CAD build for the part. Positions are in the model's coordinates, mm. Give positions to 0.01 mm unless a question says otherwise; leave off trailing zeros. Loops run counter-clockwise (first coordinate to the right, second up) from the corner with the lowest first, then second, coordinate; pieces in that order, holes last.
Item 1: Probe probe 1 along Y at (x, z) = (-1, 200); probe 2 along X at (y, z) = (-3.5, 490.5); probe 3 along X at (y, z) = (23, 372). List the from-to ranges inside material, lowest first.
Item 2: Saw through at A-A on y = -4. Give the cut face in (x, z).
Item 3: Drop flat-ended pins along their axis: P1, Ø3, axis at x = 8, z = 513, coming from the +Y side; P2, Ø8, axis at x = 0, z = 31.75, coming from the -Y side; P3, Ø4.5, axis at x = 0, z = 539.75, coming from the -Y side. Give the stop position or say it passes through.
from build123d import *

# Parameters (mm, degrees)
EXTRUDE_THIN1_DEPTH               = 571.5
F_10_CLEARANCE_HOLE1_D            = 5.1054
F_3_16_0_195_DIAMETER_HOLE1_D     = 4.953
F_3_16_0_195_DIAMETER_HOLE1_DEPTH = 1.5875


with BuildPart() as part:
    # Sketch1 → Extrude-Thin1 (new body)
    with BuildSketch(Plane.XY):
        with BuildLine():
            Line((-12.7, 19.05), (-12.7, -19.05))
            ThreePointArc((-12.7, -19.05), (-10.840128061, -23.540128061), (-6.35, -25.4))
            Line((-6.35, -25.4), (6.35, -25.4))
            ThreePointArc((6.35, -25.4), (10.840128061, -23.540128061), (12.7, -19.05))
            Line((12.7, -19.05), (12.7, 19.05))
            ThreePointArc((12.7, 19.05), (10.840128061, 23.540128061), (6.35, 25.4))
            Line((6.35, 25.4), (-6.35, 25.4))
            ThreePointArc((-6.35, 25.4), (-10.840128061, 23.540128061), (-12.7, 19.05))
        make_face()
        with BuildLine():
            Line((-11.1125, 19.05), (-11.1125, -19.05))
            ThreePointArc((-11.1125, -19.05), (-9.717596045, -22.417596045), (-6.35, -23.8125))
            Line((-6.35, -23.8125), (6.35, -23.8125))
            ThreePointArc((6.35, -23.8125), (9.717596045, -22.417596045), (11.1125, -19.05))
            Line((11.1125, -19.05), (11.1125, 19.05))
            ThreePointArc((11.1125, 19.05), (9.717596045, 22.417596045), (6.35, 23.8125))
            Line((6.35, 23.8125), (-6.35, 23.8125))
            ThreePointArc((-6.35, 23.8125), (-9.717596045, 22.417596045), (-11.1125, 19.05))
        make_face(mode=Mode.SUBTRACT)
    extrude(amount=EXTRUDE_THIN1_DEPTH)

    # #10 Clearance Hole1 (through all)
    with Locations(Plane(origin=(0, 25.4, 565.15), x_dir=(0, 0, 1), z_dir=(0, 1, 0))):
        with Locations((0, 0), (-558.8, 0), (-533.4, 0), (-508, 0), (-25.4, 0), (-50.8, 0)):
            Hole(F_10_CLEARANCE_HOLE1_D / 2)

    # 3/16 (0.195) Diameter Hole1
    with Locations(Plane(origin=(0, 25.4, 0), x_dir=(1, 0, 0), z_dir=(0, 1, 0))):
        with Locations((-3.175, -82.55), (3.175, -107.95), (-3.175, -133.35), (3.175, -158.75), (-3.175, -184.15), (3.175, -209.55), (-3.175, -234.95), (3.175, -260.35), (-3.175, -285.75), (3.175, -311.15), (-3.175, -336.55), (3.175, -361.95), (-3.175, -387.35), (3.175, -412.75), (-3.175, -438.15), (3.175, -463.55), (-3.175, -488.95)):
            Hole(F_3_16_0_195_DIAMETER_HOLE1_D / 2, depth=F_3_16_0_195_DIAMETER_HOLE1_DEPTH)


solid = part.part
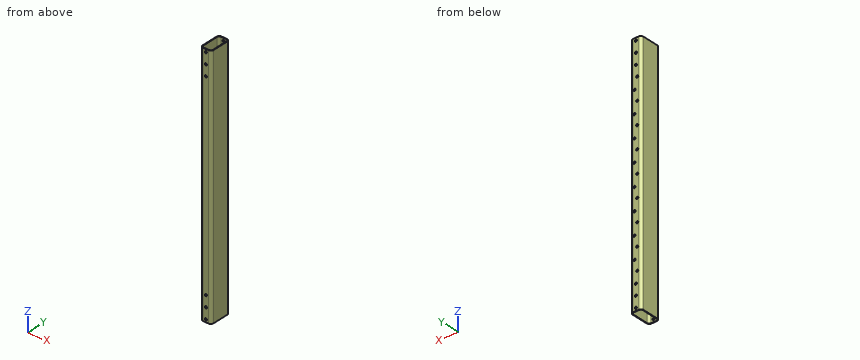
Results below:
1. probe 1: y = -25.4 to -23.81, 23.81 to 25.4
1. probe 2: x = -12.7 to -11.11, 11.11 to 12.7
1. probe 3: x = -11.32 to -9.01, 9.01 to 11.32
2. outline: (-12.7, 0) - (-11.11, 0) - (-11.11, 571.5) - (-12.7, 571.5) - close; (11.11, 0) - (12.7, 0) - (12.7, 571.5) - (11.11, 571.5) - close
3. P1: stops at y = 25.4
3. P2: stops at y = -25.4
3. P3: passes through
